```python
from build123d import *

# Parameters (mm, degrees)
F0_R     = 45.5439388368
F1_DEPTH = 139.7
F2_T     = 2.032
F5_D     = 6.35
F6_D     = 6.35
F7_D     = 6.35


# Not quite as in the source:
# - a fillet or chamfer that OpenCascade refuses, or shapes differently, is made with other operations: its cross-section is extruded or revolved along the edge and cut away or added


with BuildPart() as f1:
    # F0 (on Top) → F1 (new body)
    with BuildSketch(Plane.XY):
        Circle(F0_R)
    extrude(amount=-F1_DEPTH)

    # F2
    f2_openings = [f1.faces().sort_by_distance(p)[0] for p in [
        (0, 0, 0),
    ]]
    offset(amount=F2_T, openings=f2_openings, kind=Kind.INTERSECTION)

    # F3: fillet of radius 5.08 on 1 edges, made by hand

    # F3_s1 → F3_t2 (revolve, cut)
    with BuildSketch(Plane.XZ):
        with BuildLine():
            ThreePointArc((47.5759388368, -136.652), (46.0880412852, -140.2441024484), (42.4959388368, -141.732))
            Line((42.4959388368, -141.732), (47.5759388368, -141.732))
            Line((47.5759388368, -141.732), (47.5759388368, -136.652))
        make_face()
    revolve(axis=Axis((0, 0, -141.732), (0, 0, 1)), mode=Mode.SUBTRACT)

    # F5 (through all)
    with Locations(Plane(origin=(0, 0, -141.732), x_dir=(1, 0, 0), z_dir=(0, 0, -1))):
        with Locations((-8.5982947547, 6.4940573648), (-8.1184855662, 21.5309672058), (-14.8330600932, 26.4003239572), (-7.0802457631, 36.3871436566), (-26.5492741019, 24.3456372991), (-23.826636374, 16.2156112492), (-21.2479694184, 6.4940573648), (-33.2053042948, 4.1952142492)):
            Hole(F5_D / 2)

    # F6 (through all)
    with Locations(Plane(origin=(0, 0, -141.732), x_dir=(1, 0, 0), z_dir=(0, 0, -1))):
        with Locations((8.5982947547, 6.4940573648), (21.2479694184, 6.4940573648), (33.2053042948, 4.1952142492), (8.1184855662, 21.5309672058), (14.8330600932, 26.4003239572), (7.0802457631, 36.3871436566), (23.826636374, 16.2156112492), (26.5492741019, 24.3456372991)):
            Hole(F6_D / 2)

    # F7 (through all)
    with Locations(Plane(origin=(0, 0, -141.732), x_dir=(1, 0, 0), z_dir=(0, 0, -1))):
        with Locations((-33.2053042948, -4.1952142492), (-8.5982947547, -6.4940573648), (-21.2479694184, -6.4940573648), (-8.1184855662, -21.5309672058), (-14.8330600932, -26.4003239572), (-7.0802457631, -36.3871436566), (-26.5492741019, -24.3456372991), (-23.826636374, -16.2156112492), (8.5982947547, -6.4940573648), (33.2053042948, -4.1952142492), (21.2479694184, -6.4940573648), (23.826636374, -16.2156112492), (26.5492741019, -24.3456372991), (14.8330600932, -26.4003239572), (8.1184855662, -21.5309672058), (7.0802457631, -36.3871436566)):
            Hole(F7_D / 2)


solid = f1.part
```
Here's how the part is built. I have some questions about the finished solid (model axes, mm). A direction names the side the tool comes from. Coordinates: 2 decimals unless noted, no trailing zeros. Order: outer loops, then holes, each group sorted by start corner. A loop starts at its lowest first (then second) coordinate and runs counter-clockwise, first axis right, second up. Notation, with made-up numbers: (81.25, -31) - (126.25, -31) arc R27 ccw to (126.25, 3) - close; hole circle Ø5 at (66.25, -13). An arc over 180 degrees is marked (long way). One line per question, with ' | ' between items.
(1) If we mould it in two halves opening along X, with no side actions, what happens to faces 3 (the cylindrical face through (-10.314, -46.445, -67.369)), 4 (the flat face through (-1, 1, -141.732)), 5 (the cylindrical face through (20.894, -15, -140.702)), 6 (the cylindrical face through (5.57, 5.54, -140.7))? For each: pulls with the +X half, pulls with the -X half, needs draft (parallel to the pull), parting line crosses it, or undercut.
Report:
face 3: parting line crosses it | face 4: needs draft | face 5: undercut | face 6: undercut
(2) Will these pins go through, and if not, where does the flat tip stop? pin 1 (10 mm diameter, centred on x = 8.6, y = -6.49, fed in from -Z); pin 2 (1.5 mm diameter, centred on x = 5.5, z = -63, fed in from -Y); pin 3 (10 mm diameter, centred on x = 8.6, y = 6.49, fed in from +Z); pin 4 (6 mm diameter, centred on y = 25, z = -45, fed in from -X).
Report:
pin 1: stops at z = -141.73 | pin 2: stops at y = -47.34 | pin 3: stops at z = -139.7 | pin 4: stops at x = -42.18
(3) Suppose I cut it at C-C on x = 15.5. State how many separate pieces and enclosed holes the cut face has, and give its area (3 significant figures).
Report:
separate pieces: 3 | enclosed holes: 0 | area: 748 mm2
(4) Suppose I cut it at A-A on x = 0. List the corners of the cut face in (y, z) for me, and give its area (3 significant figures).
Report:
outline: (-47.58, -136.65) arc R5.08 ccw to (-42.5, -141.73) - (42.5, -141.73) arc R5.08 ccw to (47.58, -136.65) - (47.58, 0) - (45.54, 0) - (45.54, -139.7) - (-45.54, -139.7) - (-45.54, 0) - (-47.58, 0) - close | area: 750 mm2
(5) If I drill on L1, parallel to Z at x = 9, y = 3; L2, parallel to Y at x = 17, z = -42 (3 decimals); L3, parallel to X at y = 26.5, z = -75, over which ranges is the centre line in solid material (lowest first)?
Report:
L1: z = -141.73 to -139.7 | L2: y = -44.435 to -42.252, 42.252 to 44.435 | L3: x = -39.51 to -37.04, 37.04 to 39.51
(6) For faces 1 (the cylindrical face through (5.665, -5.278, -140.702)), 2 (the flat face through (-1, 1, -139.7)), which set-ups out of +Z, -Z, +X, -X, +Y, -Y let a thin tool reach every point of the face, with its end or its side?
Report:
face 1: +Z, -Z | face 2: +Z
(7) Suppose I cut it at B-B on z = -89. List the corners of the cut face in (x, y) for me.
Report:
outline: circle Ø95.15 at (0, 0); hole circle Ø91.09 at (0, 0)
